Drawing for the job (mm, zero at the part's lowest x, y, z). A direction names the side the tool comes from. Give positions to 0.01 mm unless a question says otherwise; leave off trailing zeros. Write each loop counter-clockwise with the first axis right and the second up, starting at its lowest first coordinate (ties: lowest second). Pieces come first, ordered by that corner, then holes.
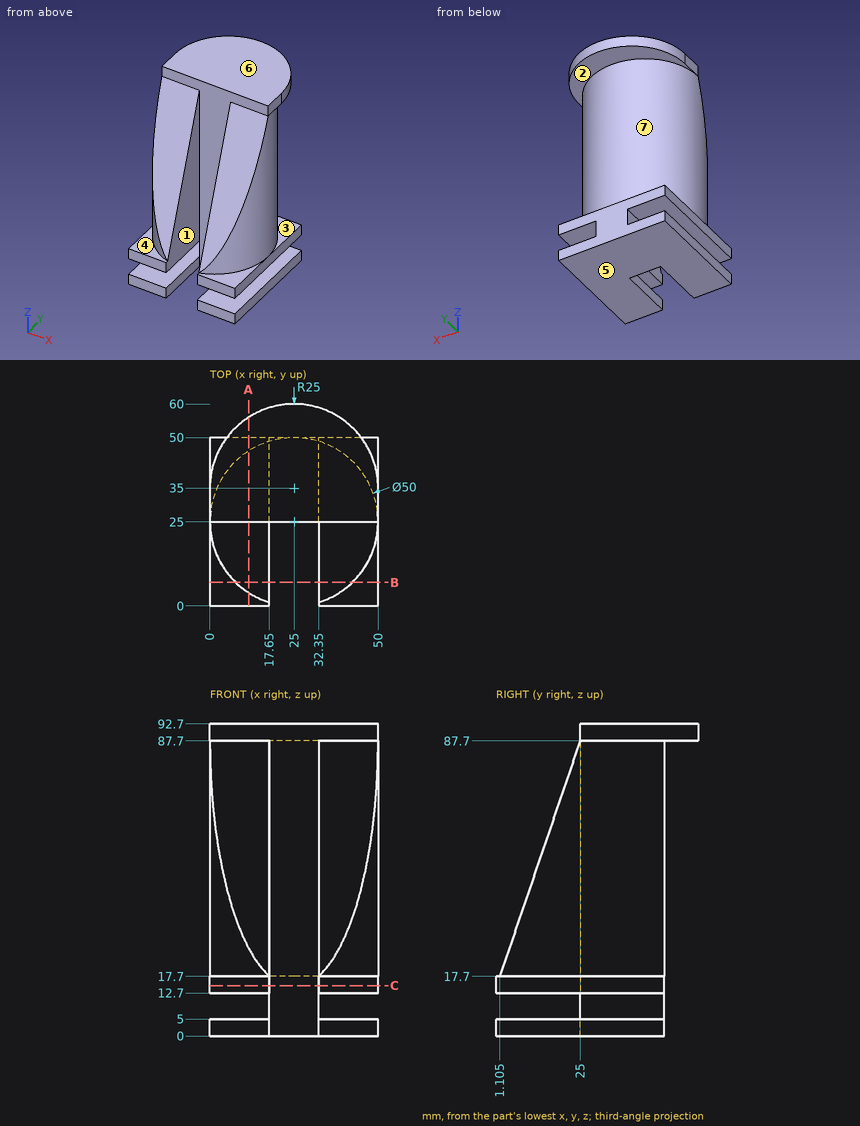
1. Pin check, flat tips, straight feed: P1, Ø7.5, axis at y = 18.5, z = 60, coming from the -X side; P2, Ø3, axis at y = 18, z = 58, coming from the -X side; P3, Ø5, axis at y = 44.5, z = 75.5, coming from the -X side. Stop position of each tip, or through.
Calculated:
P1: stops at x = 0.15
P2: stops at x = 0.61
P3: stops at x = 6.67
2. Pull direction Z, two halves, no side cores. Call the marked faces 5, 6 and 7: +Z half, -Z half, draft (parallel to the pull), parting line (faces both ways), or undercut.
Calculated:
face 5: -Z half
face 6: +Z half
face 7: undercut
3. Slice it at C-C, the plane z = 15. Write the cut outline in (x, y).
Calculated:
outline: (0, 0) - (17.65, 0) - (17.65, 25) - (32.35, 25) - (32.35, 0) - (50, 0) - (50, 50) - (0, 50) - close
4. Which spindle directions (+Z, -Z, +X, -X, +Y, -Y) get a long thin tool onto all of the face, cutting with end or side? Do the marked faces 1, 2, 3 and 4. Say none if no direction does.
Calculated:
face 1: +Z, -Z, -Y
face 2: +Y
face 3: +X, +Y
face 4: +Z, -X, -Y
5. Slice it at A-A, the plane x = 11.5. Write the cut outline in (y, z), and give its area (3 significant figures).
Calculated:
outline: (0, 0) - (50, 0) - (50, 5) - (0, 5) - close; (0, 12.7) - (50, 12.7) - (50, 17.7) - (46.04, 17.7) - (46.04, 87.7) - (56.04, 87.7) - (56.04, 92.7) - (25, 92.7) - (25, 87.7) - (3.96, 26.06) - (3.96, 17.7) - (0, 17.7) - close
area: 2,950 mm2
6. Probe probe 1 along Z at (x, y) = (15, 35); probe 2 along X at (y, z) = (40, 6.5); probe 3 along Y at (x, z) = (25, 32.5). List the from-to ranges inside material, lowest first.
Calculated:
probe 1: z = 0 to 5, 12.7 to 92.7
probe 2: x = 17.65 to 32.35
probe 3: y = 25 to 50
7. Slice it at B-B, the plane y = 7. Write the cut outline in (x, z).
Calculated:
outline: (0, 0) - (17.65, 0) - (17.65, 5) - (0, 5) - close; (0, 12.7) - (17.65, 12.7) - (17.65, 34.97) - (7.65, 34.97) - (7.65, 17.7) - (0, 17.7) - close; (32.35, 0) - (50, 0) - (50, 5) - (32.35, 5) - close; (32.35, 12.7) - (50, 12.7) - (50, 17.7) - (42.35, 17.7) - (42.35, 34.97) - (32.35, 34.97) - close
